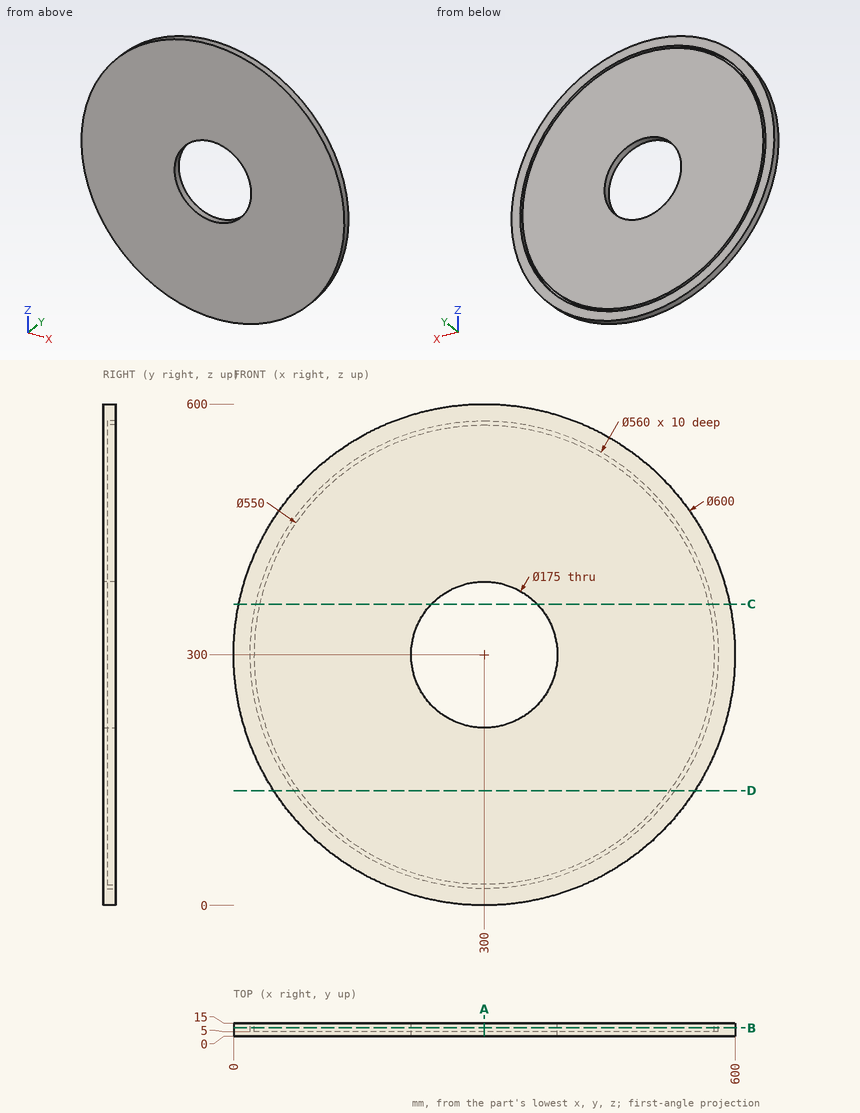
Geometry: see drawing. Coordinates: mm, zero at the bounding-box minimum. Round coordinates to 2 decimals unless told otherwise and drop trailing zeros. Write each loop counter-clockwise with the first axis right and the second up, starting at its lowest first coordinate (ties: lowest second). Pieces come first, ordered by that corner, then holes.
Item 1: Pin query (flat end, axial travel): P1, Ø8, axis at y = 4.5, z = 146.5, coming from the +X side; P2, Ø3, axis at x = 191, y = 6.5, coming from the +Z side. Return the tip coordinate at first contact, or that it passes through.
Item 2: Section query D-D (z = 137.5). Return loops of the section in (x, y).
Item 3: Material intervals for L1, parallel to X at y = 6.5, z = 300; L2, parallel to Z at x = 80, y = 11.5; L3, parallel to Z at x = 236.5, y = 7.75, sorted ascending.
Item 4: Section query B-B (y = 9.75). Return loops of the section in (x, z).
Item 5: Section query A-A (x = 300). Return loops of the section in (y, z), plus the area to 4 significant figures.
Item 6: Section query C-C (z = 360.5). Return loops of the section in (x, y).
Completed:
1. P1: stops at x = 560.1
1. P2: stops at z = 580.08
2. outline: (47.82, 0) - (552.18, 0) - (552.18, 15) - (528.02, 15) - (528.02, 5) - (521.85, 5) - (521.85, 15) - (78.15, 15) - (78.15, 5) - (71.98, 5) - (71.98, 15) - (47.82, 15) - close
3. L1: x = 0 to 20, 25 to 212.5, 387.5 to 575, 580 to 600
3. L2: z = 96.04 to 126.79, 135 to 465, 473.21 to 503.96
3. L3: z = 6.8 to 27.3, 32.43 to 239.8, 360.2 to 567.57, 572.7 to 593.2
4. outline: circle Ø600 at (300, 300); circle Ø550 at (300, 300); hole circle Ø560 at (300, 300); hole circle Ø175 at (300, 300)
5. outline: (0, 0) - (15, 0) - (15, 20) - (5, 20) - (5, 25) - (15, 25) - (15, 212.5) - (0, 212.5) - close; (0, 387.5) - (15, 387.5) - (15, 575) - (5, 575) - (5, 580) - (15, 580) - (15, 600) - (0, 600) - close
5. area: 6,275 mm2
6. outline: (6.16, 0) - (236.79, 0) - (236.79, 15) - (31.74, 15) - (31.74, 5) - (26.61, 5) - (26.61, 15) - (6.16, 15) - close; (363.21, 0) - (593.84, 0) - (593.84, 15) - (573.39, 15) - (573.39, 5) - (568.26, 5) - (568.26, 15) - (363.21, 15) - close
